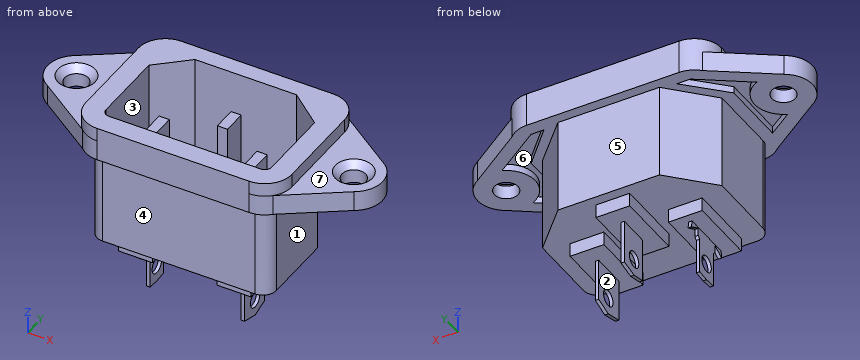
```python
from build123d import *

# Parameters (mm, degrees)
SKETCH_1_R          = 1.75
EXTRUDE_1_DEPTH     = 3
EXTRUDE_START       = 2
EXTRUDE_2_DEPTH     = 2
EXTRUDE_3_DEPTH     = 14
CUT_EXTRUDE_START   = -1
CUT_EXTRUDE_1_DEPTH = 1
CHAMFER_1_SIZE      = 1
SKETCH_6_W          = 5
SKETCH_6_H          = 10
EXTRUDE_4_DEPTH     = 2
SKETCH_7_W          = 0.5
SKETCH_7_H          = 8
EXTRUDE_5_DEPTH     = 7
SKETCH_8_R          = 1.2
CUT_EXTRUDE_2_DEPTH = 3
CUT_EXTRUDE_3_DEPTH = 3
CUT_EXTRUDE_4_DEPTH = 3
CUT_EXTRUDE_6_DEPTH = 17
SKETCH_16_W         = 5
SKETCH_16_H         = 10
EXTRUDE_7_DEPTH     = 5
SKETCH_17_W         = 1.5
SKETCH_17_H         = 3.5
EXTRUDE_8_DEPTH     = 12.5


with BuildPart() as part:
    # Sketch 1 → Extrude 1 (new body)
    with BuildSketch(Plane.XY):
        with BuildLine():
            ThreePointArc((20.928890361, -4.264902198), (23.055555556, -0.583333333), (20.928890361, 3.098235531))
            Line((20.928890361, 3.098235531), (12.38398268, 8.995093791))
            ThreePointArc((12.38398268, 8.995093791), (11.086289285, 9.862184797), (9.555555556, 10.166666667))
            Line((9.555555556, 10.166666667), (-12.944444444, 10.166666667))
            ThreePointArc((-12.944444444, 10.166666667), (-14.475178174, 9.862184797), (-15.772871569, 8.995093791))
            Line((-15.772871569, 8.995093791), (-24.387947706, 3.098235531))
            ThreePointArc((-24.387947706, 3.098235531), (-26.479451538, -0.647521096), (-24.276691296, -4.328951295))
            Line((-24.276691296, -4.328951295), (-15.772871569, -10.161760458))
            ThreePointArc((-15.772871569, -10.161760458), (-14.475178174, -11.028851463), (-12.944444444, -11.333333333))
            Line((-12.944444444, -11.333333333), (9.555555556, -11.333333333))
            ThreePointArc((9.555555556, -11.333333333), (11.086289285, -11.028851463), (12.38398268, -10.161760458))
            Line((12.38398268, -10.161760458), (20.928890361, -4.264902198))
        make_face()
        with Locations((18.805555556, -0.583333333)):
            Circle(SKETCH_1_R, mode=Mode.SUBTRACT)
        with BuildLine():
            ThreePointArc((-20.444444444, -0.583333333), (-22.194444444, -2.333333333), (-23.944444444, -0.583333333))
            ThreePointArc((-23.944444444, -0.583333333), (-22.194444444, 1.166666667), (-20.444444444, -0.583333333))
        make_face(mode=Mode.SUBTRACT)
    extrude(amount=-EXTRUDE_1_DEPTH)

    # Sketch 3 → Extrude 2 (add)
    with BuildSketch(Plane.XY.offset(EXTRUDE_START)):
        with BuildLine():
            Line((-12.944444444, 10.166666667), (9.555555556, 10.166666667))
            ThreePointArc((9.555555556, 10.166666667), (12.38398268, 8.995093791), (13.555555556, 6.166666667))
            Line((13.555555556, 6.166666667), (13.555555556, -7.333333333))
            ThreePointArc((13.555555556, -7.333333333), (12.38398268, -10.161760458), (9.555555556, -11.333333333))
            Line((9.555555556, -11.333333333), (-12.944444444, -11.333333333))
            ThreePointArc((-12.944444444, -11.333333333), (-15.772871569, -10.161760458), (-16.944444444, -7.333333333))
            Line((-16.944444444, -7.333333333), (-16.944444444, 6.166666667))
            ThreePointArc((-16.944444444, 6.166666667), (-15.772871569, 8.995093791), (-12.944444444, 10.166666667))
        make_face()
    extrude(amount=-EXTRUDE_2_DEPTH)

    # Sketch 4 → Extrude 3 (add)
    with BuildSketch(Plane(origin=(0, 0, -3), x_dir=(-1, 0, 0), z_dir=(0, 0, -1))):
        with BuildLine():
            Line((-5.805555556, 8.666666667), (9.194444444, 8.666666667))
            Line((9.194444444, 8.666666667), (14.979451538, 2.666666667))
            Line((14.979451538, 2.666666667), (14.979451538, -7.833333333))
            ThreePointArc((14.979451538, -7.833333333), (14.393665101, -9.247546896), (12.979451538, -9.833333333))
            Line((12.979451538, -9.833333333), (-9.555555556, -9.833333333))
            ThreePointArc((-9.555555556, -9.833333333), (-10.969769118, -9.247546896), (-11.555555556, -7.833333333))
            Line((-11.555555556, -7.833333333), (-11.555555556, 2.666666667))
            Line((-11.555555556, 2.666666667), (-5.805555556, 8.666666667))
        make_face()
    extrude(amount=EXTRUDE_3_DEPTH)

    # Sketch 5 → Cut-Extrude 1 (cut)
    with BuildSketch(Plane(origin=(0, 0, -3), x_dir=(-1, 0, 0), z_dir=(0, 0, -1)).offset(CUT_EXTRUDE_START)):
        with BuildLine():
            Line((-17.143050828, 3.367976899), (-10.046994094, 8.202368214))
            Line((-10.046994094, 8.202368214), (-8.140923226, 8.202368214))
            Line((-8.140923226, 8.202368214), (-13.112857934, 2.867546546))
            Line((-13.112857934, 2.867546546), (-13.112857934, -7.3554747))
            Line((-13.112857934, -7.3554747), (-17.143050828, -4.534643565))
            ThreePointArc((-17.143050828, -4.534643565), (-14.518741526, -0.583333333), (-17.143050828, 3.367976899))
        make_face()
        with BuildLine():
            Line((20.535362375, 3.367976899), (13.514232587, 8.202368214))
            Line((13.514232587, 8.202368214), (11.503497241, 8.202368214))
            Line((11.503497241, 8.202368214), (16.838318908, 2.867546546))
            Line((16.838318908, 2.867546546), (16.838318908, -7.028531022))
            Line((16.838318908, -7.028531022), (20.535362375, -4.534643565))
            ThreePointArc((20.535362375, -4.534643565), (17.908956624, -0.583333333), (20.535362375, 3.367976899))
        make_face()
    extrude(amount=CUT_EXTRUDE_1_DEPTH, mode=Mode.SUBTRACT)

    # Chamfer 1
    chamfer_1_edges = [part.edges().sort_by_distance(p)[0] for p in [
        (17.055555556, -0.583333333, 0),
    ]]
    chamfer(chamfer_1_edges, length=CHAMFER_1_SIZE)

    # Chamfer 2: read off the stored shape, not the designer's step
    # Chamfer 2 outline → Chamfer 2 (revolve, cut)
    with BuildSketch(Plane(origin=(-22.194444444, -0.583333333, 0), x_dir=(1, 0, 0), z_dir=(0, -1, 0))):
        Polygon((1.75, 0), (1.75, -1), (2.75, 0), align=None)
    revolve(axis=Axis((-22.194444444, -0.583333333, 0), (0, 0, 1)), mode=Mode.SUBTRACT)

    # Sketch 6 → Extrude 4 (add)
    with BuildSketch(Plane(origin=(0, 0, -17), x_dir=(-1, 0, 0), z_dir=(0, 0, -1))):
        with Locations((-5.555555556, -3.333333333)):
            Rectangle(SKETCH_6_W, SKETCH_6_H)
        with Locations((1.444444444, 2.166666667)):
            Rectangle(SKETCH_6_W, SKETCH_6_H)
        with Locations((8.979451538, -3.333333333)):
            Rectangle(SKETCH_6_W, SKETCH_6_H)
    extrude(amount=EXTRUDE_4_DEPTH)

    # Sketch 7 → Extrude 5 (add, symmetric)
    with BuildSketch(Plane(origin=(0, 0, -19), x_dir=(-1, 0, 0), z_dir=(0, 0, -1))):
        with Locations((-5.555555556, -3.333333333)):
            Rectangle(SKETCH_7_W, SKETCH_7_H)
        with Locations((1.444444444, 2.166666667)):
            Rectangle(SKETCH_7_W, SKETCH_7_H)
        with Locations((8.979451538, -3.333333333)):
            Rectangle(SKETCH_7_W, SKETCH_7_H)
    extrude(amount=EXTRUDE_5_DEPTH, both=True)

    # Sketch 8 → Cut-Extrude 2 (cut)
    with BuildSketch(Plane.ZY.offset(9.229451538)):
        Polygon((-26, 0.666666667), (-26, -3.333333333), (-25.852859053, -1.583646996), (-20.667626654, -1.583646996), (-20.281780656, -1.197800999), (-19.159176422, -1.197800999), (-20.028349255, 0.515685465), (-19, 0.381345072), (-19, 0.666666667), align=None)
        Polygon((-25.852859053, -5.08301967), (-26, -3.333333333), (-26, -7.333333333), (-19, -7.333333333), (-19, -7.048011738), (-20.028349255, -7.182352132), (-19.159176422, -5.468865668), (-20.281780656, -5.468865668), (-20.667626654, -5.08301967), align=None)
        with Locations(Location((-23.476723057, -3.333333333, 0), (0, 0, 270))):
            Circle(SKETCH_8_R)
    extrude(amount=-CUT_EXTRUDE_2_DEPTH, mode=Mode.SUBTRACT)

    # Sketch 11 → Cut-Extrude 3 (cut)
    with BuildSketch(Plane.ZY.offset(1.694444444)):
        with BuildLine():
            ThreePointArc((-24.7, 2.166666667), (-23.5, 0.966666667), (-22.3, 2.166666667))
            Line((-22.3, 2.166666667), (-24.7, 2.166666667))
        make_face()
        with BuildLine():
            Line((-24.7, 2.166666667), (-22.3, 2.166666667))
            ThreePointArc((-22.3, 2.166666667), (-23.5, 3.366666667), (-24.7, 2.166666667))
        make_face()
        Polygon((-25.500216553, 4.64880104), (-19, 4.64880104), (-19, 6.166666667), (-26, 6.166666667), (-26, 4.64880104), (-26, 2.166666667), align=None)
        Polygon((-19, -1.833333333), (-19, 0), (-25.500216553, 0), (-26, 2.166666667), (-26, 0), (-26, -1.833333333), align=None)
    extrude(amount=-CUT_EXTRUDE_3_DEPTH, mode=Mode.SUBTRACT)

    # Sketch 12 → Cut-Extrude 4 (cut)
    with BuildSketch(Plane.ZY.offset(-5.305555556)):
        Polygon((-25.256261819, -0.896417806), (-19, -0.896417806), (-19, 0.666666667), (-26, 0.666666667), (-26, -0.896417806), (-26, -3.333333333), align=None)
        Polygon((-19, -7.333333333), (-19, -6.035631996), (-25.256261819, -6.035631996), (-26, -3.333333333), (-26, -6.035631996), (-26, -7.333333333), align=None)
        with BuildLine():
            ThreePointArc((-24.7, -3.333333333), (-23.5, -4.533333333), (-22.3, -3.333333333))
            Line((-22.3, -3.333333333), (-24.7, -3.333333333))
        make_face()
        with BuildLine():
            Line((-24.7, -3.333333333), (-22.3, -3.333333333))
            ThreePointArc((-22.3, -3.333333333), (-23.5, -2.133333333), (-24.7, -3.333333333))
        make_face()
    extrude(amount=-CUT_EXTRUDE_4_DEPTH, mode=Mode.SUBTRACT)

    # Sketch 15 → Cut-Extrude 6 (cut)
    with BuildSketch(Plane.XY.offset(2)):
        with BuildLine():
            Line((-9.444444444, 7.666666667), (5.555555556, 7.666666667))
            Line((5.555555556, 7.666666667), (10.555555556, 3.666666667))
            Line((10.555555556, 3.666666667), (10.555555556, -7.333333333))
            ThreePointArc((10.555555556, -7.333333333), (10.262662337, -8.040440115), (9.555555556, -8.333333333))
            Line((9.555555556, -8.333333333), (-12.944444444, -8.333333333))
            ThreePointArc((-12.944444444, -8.333333333), (-13.651551226, -8.040440115), (-13.944444444, -7.333333333))
            Line((-13.944444444, -7.333333333), (-13.944444444, 3.666666667))
            Line((-13.944444444, 3.666666667), (-9.444444444, 7.666666667))
        make_face()
    extrude(amount=-CUT_EXTRUDE_6_DEPTH, mode=Mode.SUBTRACT)

    # Sketch 16 → Extrude 7 (add)
    with BuildSketch(Plane(origin=(0, 0, -19), x_dir=(-1, 0, 0), z_dir=(0, 0, -1))):
        with Locations((8.979451538, -3.333333333)):
            Rectangle(SKETCH_16_W, SKETCH_16_H)
        with Locations((1.444444444, 2.166666667)):
            Rectangle(SKETCH_16_W, SKETCH_16_H)
        with Locations((-5.555555556, -3.333333333)):
            Rectangle(SKETCH_16_W, SKETCH_16_H)
    extrude(amount=-EXTRUDE_7_DEPTH)

    # Sketch 17 → Extrude 8 (add)
    with BuildSketch(Plane.XY.offset(-14)):
        with Locations((-8.961393916, -2.773412546)):
            Rectangle(SKETCH_17_W, SKETCH_17_H)
        with Locations((-1.478668657, 2.665013022)):
            Rectangle(SKETCH_17_W, SKETCH_17_H)
        with Locations((5.641966267, -3.00690977)):
            Rectangle(SKETCH_17_W, SKETCH_17_H)
    extrude(amount=EXTRUDE_8_DEPTH)


solid = part.part
```
Here's how the part is built. I have some questions about the finished solid (model axes, mm). Face numbers are marked on the shaded views. A direction names the side the tool comes from. Coordinates: 2 decimals unless noted, no trailing zeros. Order: outer loops, then holes, each group sorted by start corner. A loop starts at its lowest first (then second) coordinate and runs counter-clockwise, first axis right, second up.
1) I need wall thicknesses on line 1 (X direction, y = -0.5, z = -17.75); line 2 (Y direction, x = -1.4, z = -23.5); line 3 (X direction, y = 1, z = -6). Which ranges of each line are inside material? Lowest first, please.
2) Imagine slicing it at B-B on z = -18.25. List the corners of the cut face in (x, y) for me, and give its area (3 significant figures).
3) Imagine slicing it at A-A on z = -7.25. List the corners of the cut face in (x, y) for me.
4) We'd pull the mould along Y, two halves only. Please class the marked faces 5, 6 and 7: +Y half, -Y half, draft (parallel to the pull), parting line (faces both ways), or undercut.
5) Will these pins go through, and if not, where does the flat tip stop? pin 1 (8 mm diameter, centred on x = 2, y = 1.5, fed in from +Z); pin 2 (5 mm diameter, centred on x = 14, y = -6, fed in from -Z); pin 3 (4 mm diameter, centred on y = -2, z = -5.5, fed in from +X); pin 4 (8 mm diameter, centred on x = 6, y = -7, fed in from -Z).
6) Which directions (+Z, -Z, +X, -X, +Y, -Y) give clear straight access to the entire face, cutting with the end or side of a thin tool? Please do the marked faces 1, 2, 3 and 4.
Response values:
1. line 1: x = -11.48 to -6.48, -3.94 to 1.06, 3.06 to 8.06
1. line 2: y = 0 to 0.97, 3.37 to 4.65
1. line 3: x = -14.98 to -13.94, -2.23 to -0.73, 10.56 to 11.56
2. outline: (-11.48, -8.33) - (-6.48, -8.33) - (-6.48, 1.67) - (-11.48, 1.67) - close; (-3.94, -2.83) - (1.06, -2.83) - (1.06, 7.17) - (-3.94, 7.17) - close; (3.06, -8.33) - (8.06, -8.33) - (8.06, 1.67) - (3.06, 1.67) - close
2. area: 150 mm2
3. outline: (-14.98, -7.83) arc R2 ccw to (-12.98, -9.83) - (9.56, -9.83) arc R2 ccw to (11.56, -7.83) - (11.56, 2.67) - (5.81, 8.67) - (-9.19, 8.67) - (-14.98, 2.67) - close; (-9.71, -4.52) - (-8.21, -4.52) - (-8.21, -1.02) - (-9.71, -1.02) - close; (-2.23, 0.92) - (-0.73, 0.92) - (-0.73, 4.42) - (-2.23, 4.42) - close; (4.89, -4.76) - (6.39, -4.76) - (6.39, -1.26) - (4.89, -1.26) - close; hole (-13.94, -7.33) arc R1 ccw to (-12.94, -8.33) - (9.56, -8.33) arc R1 ccw to (10.56, -7.33) - (10.56, 3.67) - (5.56, 7.67) - (-9.44, 7.67) - (-13.94, 3.67) - close
4. face 5: +Y half
4. face 6: undercut
4. face 7: draft
5. pin 1: stops at z = -1.5
5. pin 2: stops at z = -17
5. pin 3: stops at x = 11.56
5. pin 4: stops at z = -26
6. face 1: -Z, +X, +Y, -Y
6. face 2: -Z, +Y, -Y
6. face 3: +Z
6. face 4: -Z, +X, -X, -Y
